Input: part model. Units: mm. Frame: model coordinates. A direction names the side the tool comes from. Give positions to 0.01 mm unless a question says otherwise; leave off trailing zeros. Loops run counter-clockwise (first coordinate to the right, second up) from the corner with the lowest first, then second, coordinate; pieces in that order, holes last. Notation, with made-up numbers: (39, -5) -> (66, -5) arc R20 cw to (66, 15) -> close; hole circle Ø7 at (-28, 55.5). An arc over 180 degrees is marked (long way). One line per question, with ' | ' between items.
Autodesk Inventor part; units mm, degrees
ref_plane "YZ Plane" through (0, 0, 0) normal (1, 0, 0) x (0, 1, 0)
ref_plane "XZ Plane" through (0, 0, 0) normal (0, 1, 0) x (-1, 0, 0)
ref_plane "XY Plane" through (0, 0, 0) normal (0, 0, 1) x (1, 0, 0)
sketch "Skizze1" plane through (0, 0, 0) normal (0, 1, 0) x (-1, 0, 0)
  line L0 (0, 0) -> (-50, 0)
  line L1 (-50, 0) -> (-50, 25)
  line L2 (-50, 25) -> (0, 25)
  line L3 (0, 25) -> (0, 0)
  line L4 (0, 0) -> (-25, 0)
  line L5 (-25, 0) -> (-25, -25)
  line L6 (-25, -25) -> (0, -25)
  line L7 (0, -25) -> (0, 0)
  dimension "d0" = 50
  dimension "d1" = 25
  dimension "d2" = 25
  dimension "d3" = 25
extrude "Extrusion1" add sketch "Skizze1" along normal blind 10
sketch "Skizze2" plane through (50, 0, 25) normal (1, 0, 0) x (0, 0, -1)
  line L0 (25, 0) -> (25, 10)
  line L1 (25, 7) -> (5, 7)
  line L2 (5, 7) -> (5, 3)
  line L3 (5, 3) -> (25, 3)
  line L4 (25, 3) -> (25, 7)
  line L5 (0, 10) -> (25, 10)
  line L6 (0, 0) -> (25, 0)
  point P0 (12.5, 10)
  dimension "d6" = 3
  dimension "d7" = 3
  dimension "d8" = 20
extrude "Extrusion2" cut sketch "Skizze2" against normal blind 45
sketch "Skizze3" plane through (25, 0, -25) normal (0, 0, -1) x (-1, 0, 0)
  line L0 (0, 3) -> (20, 3)
  line L1 (20, 7) -> (20, 3)
  line L2 (0, 3) -> (20, 3)
  line L3 (20, 3) -> (20, 7)
  line L4 (20, 7) -> (0, 7)
  line L5 (0, 7) -> (0, 3)
  point P0 (25, 0)
extrude "Extrusion3" cut sketch "Skizze3" against normal blind 45
sketch "Skizze4" plane through (0, 10, 0) normal (0, 1, 0) x (1, 0, 0)
  line L0 (50, -20) -> (5, -20)
  line L1 (25, 0) -> (5, 0)
  line L2 (5, 0) -> (5, -20)
  line L3 (5, -20) -> (25, -20)
  line L4 (25, -20) -> (25, 0)
  line L5 (5, -20) -> (35, -20)
  line L6 (35, -20) -> (35, 10)
  line L7 (35, 10) -> (5, 10)
  line L8 (5, 10) -> (5, -20)
  circle A0 centre (20, -5) radius 1.7
  point P0 (0, 0)
  dimension "d13" = 30
  dimension "d14" = 30
  dimension "d15" = 3.4
extrude "Extrusion4" cut sketch "Skizze4" against normal blind 3 contours A0
equation "\"Biegeradius\" = Stärke"
equation "\"BreiteBiegungsfreistellung\" = Stärke"
equation "\"TiefeBiegungsfreistellung\" = 0.5 * Stärke"
equation "\"GrößeEckenfreistellung\" = 4 * Stärke"
equation "\"MinimalRest\" = 2 * Stärke"
equation "\"Übergangsradius\" = Biegeradius"
equation "\"JacobiRadiusGröße\" = Biegeradius"
equation "\"Abstandsgröße\" = Stärke"
properties part number "Eckenbohren"
1. Section query C-C (y = 7.75). Output: boundary loops of the cut face in (x, z).
Determined:
outline: (0, -25) -> (25, -25) -> (25, 0) -> (50, 0) -> (50, 25) -> (0, 25) -> close; hole circle Ø3.4 at (20, 5)
2. Section query B-B (x = 20). Output: boundary loops of the cut face in (y, z), then the cut area to 3 significant figures.
Determined:
outline: (0, -25) -> (3, -25) -> (3, 20) -> (7, 20) -> (7, 6.7) -> (10, 6.7) -> (10, 25) -> (0, 25) -> close; (7, -25) -> (10, -25) -> (10, 3.3) -> (7, 3.3) -> close | area: 310 mm2
3. Section query D-D (z = -20.5). Output: boundary loops of the cut face in (x, y).
Determined:
outline: (0, 0) -> (25, 0) -> (25, 3) -> (5, 3) -> (5, 7) -> (25, 7) -> (25, 10) -> (0, 10) -> close
4. Ray query, line 1 along Z through (x, y) = (20, 9.1); line 2 along Y through (x, z) = (15.5, -3.5); line 3 along X through (y, z) = (8.05, 5). Return the intervals inside material, ascending. Write a range as from..to.
Determined:
line 1: z = -25..3.3, 6.7..25 | line 2: y = 0..3, 7..10 | line 3: x = 0..18.3, 21.7..50
5. Reachability of faces 1 (the flat face through (23, 3, 2)), 2 (the flat face through (25, 1, -12)), 3 (the flat face through (0, 5, 0)) from +Z, -Z, +X, -X, +Y, -Y: full face, straight path, thin tool, end or side. Return the list, or none.
Determined:
face 1: -Z, +X | face 2: -Z, +X, +Y, -Y | face 3: +Z, -Z, -X, +Y, -Y
6. Section query A-A (z = 5). Output: boundary loops of the cut face in (x, y).
Determined:
outline: (0, 0) -> (50, 0) -> (50, 3) -> (5, 3) -> (5, 7) -> (18.3, 7) -> (18.3, 10) -> (0, 10) -> close; (21.7, 7) -> (50, 7) -> (50, 10) -> (21.7, 10) -> close
7. Pin query (flat end, axial travel): P1, Ø2.5, axis at y = 9, z = -16.5, coming from the +X side; P2, Ø1.5, axis at x = 42, y = 2, coming from the -Z side; P3, Ø5, axis at y = 6.5, z = 19, coming from the -X side; P4, Ø1.2, axis at x = 32.5, y = 5.5, coming from the -Z side. Return the tip coordinate at first contact, or that it passes through.
Determined:
P1: stops at x = 25 | P2: stops at z = 0 | P3: stops at x = 0 | P4: stops at z = 20
8. Pull-direction query (X, two-part tool) for faces 4 (the flat face through (25, 8, -12)), 5 (the flat face through (12.7, 2.7, -25)), 6 (the cylindrical face through (21.57, 8.52, 5.65)); classes: pulls with the +X half, pulls with the -X half, needs draft (parallel to the pull), parting line crosses it, or undercut.
Determined:
face 4: pulls with the +X half | face 5: needs draft | face 6: undercut
